```python
from build123d import *

# Parameters (mm, degrees)
F1_DEPTH = 2
F2_R     = 1
F3_DEPTH = 2.001


with BuildPart() as f1:
    # F0 (on Top) → F1 (new body)
    with BuildSketch(Plane.XY):
        with BuildLine():
            ThreePointArc((4.977473, -0.474095), (4.994365, -0.237315), (5, 0))
            ThreePointArc((5, 0), (4.994365, 0.237315), (4.977473, 0.474095))
            ThreePointArc((4.977473, 0.474095), (4.755283, 1.545085), (4.305526, 2.542134))
            ThreePointArc((4.305526, 2.542134), (4.045085, 2.938926), (3.748194, 3.309236))
            ThreePointArc((3.748194, 3.309236), (2.938926, 4.045085), (1.989014, 4.587355))
            ThreePointArc((1.989014, 4.587355), (1.545085, 4.755283), (1.087233, 4.880361))
            ThreePointArc((1.087233, 4.880361), (0, 5), (-1.087233, 4.880361))
            ThreePointArc((-1.087233, 4.880361), (-1.545085, 4.755283), (-1.989014, 4.587355))
            ThreePointArc((-1.989014, 4.587355), (-2.938926, 4.045085), (-3.748194, 3.309236))
            ThreePointArc((-3.748194, 3.309236), (-4.045085, 2.938926), (-4.305526, 2.542134))
            ThreePointArc((-4.305526, 2.542134), (-4.755283, 1.545085), (-4.977473, 0.474095))
            ThreePointArc((-4.977473, 0.474095), (-5, 0), (-4.977473, -0.474095))
            ThreePointArc((-4.977473, -0.474095), (-4.755283, -1.545085), (-4.305526, -2.542134))
            ThreePointArc((-4.305526, -2.542134), (-4.045085, -2.938926), (-3.748194, -3.309236))
            ThreePointArc((-3.748194, -3.309236), (-2.938926, -4.045085), (-1.989014, -4.587355))
            ThreePointArc((-1.989014, -4.587355), (-1.545085, -4.755283), (-1.087233, -4.880361))
            ThreePointArc((-1.087233, -4.880361), (0, -5), (1.087233, -4.880361))
            ThreePointArc((1.087233, -4.880361), (1.545085, -4.755283), (1.989014, -4.587355))
            ThreePointArc((1.989014, -4.587355), (2.938926, -4.045085), (3.748194, -3.309236))
            ThreePointArc((3.748194, -3.309236), (4.045085, -2.938926), (4.305526, -2.542134))
            ThreePointArc((4.305526, -2.542134), (4.755283, -1.545085), (4.977473, -0.474095))
        make_face()
        with BuildLine():
            ThreePointArc((4.305526, 2.542134), (4.755283, 1.545085), (4.977473, 0.474095))
            ThreePointArc((4.977473, 0.474095), (5.987228, 0.940952), (6.811904, 1.687591))
            Line((6.811904, 1.687591), (6.657396, 2.163119))
            Line((6.657396, 2.163119), (6.502887, 2.638647))
            ThreePointArc((6.502887, 2.638647), (5.396847, 2.757958), (4.305526, 2.542134))
        make_face()
        with BuildLine():
            ThreePointArc((6.811904, -1.687591), (5.987228, -0.940952), (4.977473, -0.474095))
            ThreePointArc((4.977473, -0.474095), (4.755283, -1.545085), (4.305526, -2.542134))
            ThreePointArc((4.305526, -2.542134), (5.396847, -2.757958), (6.502887, -2.638647))
            Line((6.502887, -2.638647), (6.657396, -2.163119))
            Line((6.657396, -2.163119), (6.811904, -1.687591))
        make_face()
        with BuildLine():
            ThreePointArc((1.989014, 4.587355), (2.938926, 4.045085), (3.748194, 3.309236))
            ThreePointArc((3.748194, 3.309236), (4.290691, 4.28045), (4.519005, 5.369226))
            Line((4.519005, 5.369226), (4.114497, 5.663119))
            Line((4.114497, 5.663119), (3.709988, 5.957012))
            ThreePointArc((3.709988, 5.957012), (2.745054, 5.403422), (1.989014, 4.587355))
        make_face()
        with BuildLine():
            ThreePointArc((4.519005, -5.369226), (4.290691, -4.28045), (3.748194, -3.309236))
            ThreePointArc((3.748194, -3.309236), (2.938926, -4.045085), (1.989014, -4.587355))
            ThreePointArc((1.989014, -4.587355), (2.745054, -5.403422), (3.709988, -5.957012))
            Line((3.709988, -5.957012), (4.114497, -5.663119))
            Line((4.114497, -5.663119), (4.519005, -5.369226))
        make_face()
        with BuildLine():
            ThreePointArc((-1.087233, 4.880361), (0, 5), (1.087233, 4.880361))
            ThreePointArc((1.087233, 4.880361), (0.955257, 5.984962), (0.5, 7))
            Line((0.5, 7), (0, 7))
            Line((0, 7), (-0.5, 7))
            ThreePointArc((-0.5, 7), (-0.955257, 5.984962), (-1.087233, 4.880361))
        make_face()
        with BuildLine():
            ThreePointArc((0.5, -7), (0.955257, -5.984962), (1.087233, -4.880361))
            ThreePointArc((1.087233, -4.880361), (0, -5), (-1.087233, -4.880361))
            ThreePointArc((-1.087233, -4.880361), (-0.955257, -5.984962), (-0.5, -7))
            Line((-0.5, -7), (0, -7))
            Line((0, -7), (0.5, -7))
        make_face()
        with BuildLine():
            ThreePointArc((-3.748194, 3.309236), (-2.938926, 4.045085), (-1.989014, 4.587355))
            ThreePointArc((-1.989014, 4.587355), (-2.745054, 5.403422), (-3.709988, 5.957012))
            Line((-3.709988, 5.957012), (-4.114497, 5.663119))
            Line((-4.114497, 5.663119), (-4.519005, 5.369226))
            ThreePointArc((-4.519005, 5.369226), (-4.290691, 4.28045), (-3.748194, 3.309236))
        make_face()
        with BuildLine():
            ThreePointArc((-3.709988, -5.957012), (-2.745054, -5.403422), (-1.989014, -4.587355))
            ThreePointArc((-1.989014, -4.587355), (-2.938926, -4.045085), (-3.748194, -3.309236))
            ThreePointArc((-3.748194, -3.309236), (-4.290691, -4.28045), (-4.519005, -5.369226))
            Line((-4.519005, -5.369226), (-4.114497, -5.663119))
            Line((-4.114497, -5.663119), (-3.709988, -5.957012))
        make_face()
        with BuildLine():
            ThreePointArc((-4.977473, 0.474095), (-4.755283, 1.545085), (-4.305526, 2.542134))
            ThreePointArc((-4.305526, 2.542134), (-5.396847, 2.757958), (-6.502887, 2.638647))
            Line((-6.502887, 2.638647), (-6.657396, 2.163119))
            Line((-6.657396, 2.163119), (-6.811904, 1.687591))
            ThreePointArc((-6.811904, 1.687591), (-5.987228, 0.940952), (-4.977473, 0.474095))
        make_face()
        with BuildLine():
            ThreePointArc((-6.502887, -2.638647), (-5.396847, -2.757958), (-4.305526, -2.542134))
            ThreePointArc((-4.305526, -2.542134), (-4.755283, -1.545085), (-4.977473, -0.474095))
            ThreePointArc((-4.977473, -0.474095), (-5.987228, -0.940952), (-6.811904, -1.687591))
            Line((-6.811904, -1.687591), (-6.657396, -2.163119))
            Line((-6.657396, -2.163119), (-6.502887, -2.638647))
        make_face()
    extrude(amount=F1_DEPTH)

    # F2 (on face) → F3 (cut, through all)
    with BuildSketch(Plane.XY.offset(2)):
        Circle(F2_R)
    extrude(amount=-F3_DEPTH, mode=Mode.SUBTRACT)


solid = f1.part
```
For this review, take the finished solid that the model builds, in its own axes (mm). A direction names the side the tool comes from. Give positions to 0.01 mm unless a question says otherwise; leave off trailing zeros. Loops run counter-clockwise (first coordinate to the right, second up) from the corner with the lowest first, then second, coordinate; pieces in that order, holes last. Notation, with made-up numbers: M 61.25,-16.5 L 118.25,-16.5 A20 ccw 118.25,8.5 Z; hole C 48,-28.75 d6. An arc over 180 degrees is marked long. One line per item, written item: value. Start each with the question number.
Q1. Add section B-B (y = -0.75). Give the boundary of the cut face in (x, z).
Q2. Add section A-A (x = 0). Give the boundary of the cut face in (y, z).
Q3. Machinability: for faces 4 (the face through (5.97, 0.93, 0.99)), 5 (the face through (1.551, 4.753, 0.986)), 6 (the face through (-1.551, -4.753, 0.986)), which of the approach directions +Z, -Z, +X, -X, +Y, -Y give a long, thin tool a straight path to every point of the face, cutting with its end or side? Answer none if there is none.
Q4. For L1, parallel to Y at x = 0, z = 1.35; L2, parallel to Y at x = -4, z = 0.65; L3, parallel to Y at x = 6, z = 1.55, list the stretches that pass through material, from the lowest coordinate up.
Q5. Add section C-C (x = -3.25). Give the boundary of the cut face in (y, z), and give its area (3 significant figures).
Q6. Draft analysis for pull direction Y (two halves, no side actions). For faces 1 (the face through (-2.757, -5.413, 0.986)), 2 (the face through (0, 7, 1)), 3 (the face through (-6, 0.95, 0.99)), state which applies: released by +Y, released by -Y, zero draft, split by the parting line, or undercut.
Q7. Add section D-D (x = 3). Give the boundary of the cut face in (y, z).
Reply:
1. outline: M -5.66,0 L -0.66,0 L -0.66,2 L -5.66,2 Z; M 0.66,0 L 5.66,0 L 5.66,2 L 0.66,2 Z
2. outline: M -7,0 L -1,0 L -1,2 L -7,2 Z; M 1,0 L 7,0 L 7,2 L 1,2 Z
3. face 4: +Z, -Z, +X
3. face 5: +Z, -Z, +Y
3. face 6: +Z, -Z, -Y
4. L1: -7 to -1, 1 to 7
4. L2: -5.75 to -3.68, -3 to 3, 3.68 to 5.75
4. L3: -2.74 to -0.95, 0.95 to 2.74
5. outline: M -5.74,0 L 5.74,0 L 5.74,2 L -5.74,2 Z
5. area: 23.0 mm²
6. face 1: released by -Y
6. face 2: released by +Y
6. face 3: undercut
7. outline: M -5.59,0 L 5.59,0 L 5.59,2 L -5.59,2 Z
